```python
from build123d import *

# Parameters (mm, degrees)
SKETCH1_R           = 1.55
BOSS_EXTRUDE1_DEPTH = 2
CHAMFER1_SIZE       = 0.2


with BuildPart() as part:
    # Sketch1 → Boss-Extrude1 (new body)
    with BuildSketch(Plane(origin=(0, 0, 0), x_dir=(0, 0, -1), z_dir=(1, 0, 0))):
        with BuildLine():
            Line((-12, 2.5), (12, 2.5))
            ThreePointArc((12, 2.5), (14.5, 0), (12, -2.5))
            Line((12, -2.5), (-12, -2.5))
            ThreePointArc((-12, -2.5), (-14.5, 0), (-12, 2.5))
        make_face()
        with Locations((-12, 0)):
            Circle(SKETCH1_R, mode=Mode.SUBTRACT)
        with Locations((12, 0)):
            Circle(SKETCH1_R, mode=Mode.SUBTRACT)
    extrude(amount=BOSS_EXTRUDE1_DEPTH)

    # Chamfer1
    chamfer1_edges = [part.edges().sort_by_distance(p)[0] for p in [
        (0, 0, 13.55),
        (2, 0, 13.55),
        (2, 0, -14.5),
        (0, 0, -10.45),
        (2, 0, -10.45),
        (2, 2.5, 0),
        (2, 0, 14.5),
        (0, 2.5, 0),
        (0, 0, -14.5),
        (0, -2.5, 0),
        (0, 0, 14.5),
        (2, -2.5, 0),
    ]]
    chamfer(chamfer1_edges, length=CHAMFER1_SIZE)


solid = part.part
```
Could you check a few things on this model? Use its own coordinates, in mm. Coordinates: 2 decimals unless noted, no trailing zeros. Write each loop counter-clockwise with the first axis right and the second up, starting at its lowest first coordinate (ties: lowest second). Pieces come first, ordered by that corner, then holes. Notation, with made-up numbers: (68, -1) -> (74, -1) arc R20 cw to (74, 14) -> close; hole circle Ø7 at (-28, 33.25). An arc over 180 degrees is marked (long way). Return JSON: item names as keys, results as strings.
(1) Imagine slicing it at B-B, the plane x = 1.45. Please give me the cut outline in (y, z).
Numbers:
{"outline": "(-2.5, -12) arc R2.5 ccw to (2.5, -12) -> (2.5, 12) arc R2.5 ccw to (-2.5, 12) -> close; hole circle Ø3.1 at (0, -12); hole circle Ø3.1 at (0, 12)"}
(2) I need wall thicknesses on L1, parallel to Y at x = 0.9, z = -12; L2, parallel to Z at x = 1.6, y = 1.15; L3, parallel to Z at x = 1.2, y = -0.8. Which ranges of each line are inside material? Lowest first, please.
Numbers:
{"L1": "y = -2.5 to -1.55, 1.55 to 2.5", "L2": "z = -14.22 to -13.04, -10.96 to 10.96, 13.04 to 14.22", "L3": "z = -14.37 to -13.33, -10.67 to 10.67, 13.33 to 14.37"}
(3) I'm going to push a flat-ended pin straight in: pin 1 (1 mm diameter, centred on y = 1, z = 0.5, fed in from -X). Where does the tip first touch, or does it pass through?
Numbers:
{"pin 1": "stops at x = 0"}
(4) We'd pull the mould along Y, two halves only. Please class faces 1 (the flat face through (1, -2.5, 0)), 2 (the cylindrical face through (0.99, -0.94, 13.23)), 3 (the flat face through (0, 0, 0)): +Y half, -Y half, draft (parallel to the pull), parting line (faces both ways), or undercut.
Numbers:
{"face 1": "-Y half", "face 2": "undercut", "face 3": "draft"}
(5) Imagine slicing it at A-A, the plane y = 0. Please give me the cut outline in (x, z).
Numbers:
{"outline": "(0, -14.3) -> (0.2, -14.5) -> (1.8, -14.5) -> (2, -14.3) -> (2, -13.75) -> (1.8, -13.55) -> (0.2, -13.55) -> (0, -13.75) -> close; (0, -10.25) -> (0.2, -10.45) -> (1.8, -10.45) -> (2, -10.25) -> (2, 10.25) -> (1.8, 10.45) -> (0.2, 10.45) -> (0, 10.25) -> close; (0, 13.75) -> (0.2, 13.55) -> (1.8, 13.55) -> (2, 13.75) -> (2, 14.3) -> (1.8, 14.5) -> (0.2, 14.5) -> (0, 14.3) -> close"}
